Verification items for the finished model (mm, model axes). Face numbers are marked on the shaded views. A direction names the side the tool comes from. Give positions to 0.01 mm unless a question says otherwise; leave off trailing zeros. Write each loop counter-clockwise with the first axis right and the second up, starting at its lowest first coordinate (ties: lowest second). Pieces come first, ordered by that corner, then holes. Notation, with made-up numbers: (-16, -36.75) -> (31, -36.75) arc R13 cw to (31, -13.75) -> close; hole circle Ø11 at (72, 38.5). An arc over 180 degrees is marked (long way). Answer as CSV lines item,"result".
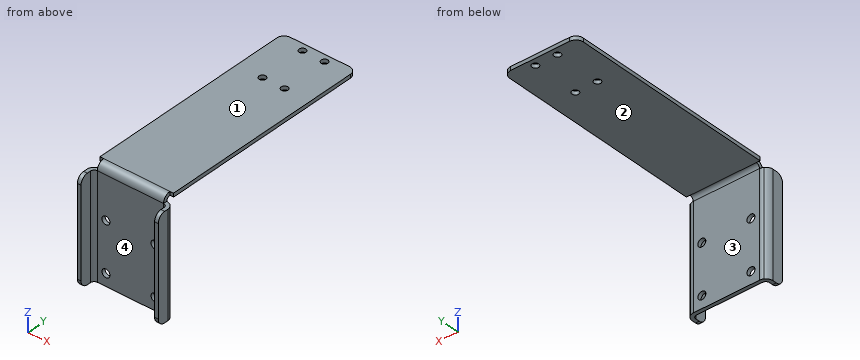
```python
from build123d import *

# Parameters (mm, degrees)
SKIZZE1_W                        = 60
SKIZZE1_H                        = 180
BASIS_BLECH1_DEPTH               = 3
KANTE_LASCHE1_STRIP_W            = 18
KANTE_LASCHE1_STRIP_H            = 3
KANTE_LASCHE1_STRIP_CUT_DEPTH    = 60
KANTE_LASCHE1_DEPTH              = 60
KANTE_LASCHE2_START              = -90.5
KANTE_LASCHE2_DEPTH              = 90.5
KANTE_LASCHE2_START_2            = -6
KANTE_LASCHE2_2_DEPTH            = 6
KANTE_LASCHE2_3_DEPTH            = 84.5
ECKE_START                       = -33
ECKE_BRECHEN1_DEPTH              = 66
ECKE_START_2                     = -3
ECKE_BRECHEN1_2_DEPTH            = 3
F_6_5_6_5_DURCHMESSER_BOHRUNG1_D = 6.5
F_5_5_5_5_DURCHMESSER_BOHRUNG1_D = 5.5


# Read off the part's stored shape, not the designer's step: Kante-Lasche2, Ecke brechen1
# Sheet-metal steps are written as plain solids
with BuildPart() as part:
    # Skizze1 → Basis-Blech1 (new body)
    with BuildSketch(Plane.XY):
        Rectangle(SKIZZE1_W, SKIZZE1_H)
    extrude(amount=-BASIS_BLECH1_DEPTH)

    # Kante-Lasche1 strip (across the edge) → Kante-Lasche1 strip cut (cut)
    with BuildSketch(Plane(origin=(30, -90, -3), x_dir=(0, 1, 0), z_dir=(-1, 0, 0))):
        with Locations((-3, -1.5)):
            Rectangle(KANTE_LASCHE1_STRIP_W, KANTE_LASCHE1_STRIP_H)
    extrude(amount=KANTE_LASCHE1_STRIP_CUT_DEPTH, mode=Mode.SUBTRACT)

    # Kante-Lasche1 section (across the edge) → Kante-Lasche1 (add)
    with BuildSketch(Plane(origin=(30, -90, -3), x_dir=(0, 1, 0), z_dir=(-1, 0, 0))):
        with BuildLine():
            Line((0, 3), (0, 87.5))
            Line((0, 87.5), (3, 87.5))
            Line((3, 87.5), (3, 3))
            ThreePointArc((3, 3), (3.878679656, 0.878679656), (6, 0))
            Line((6, 0), (6, -3))
            ThreePointArc((6, -3), (1.757359313, -1.242640687), (0, 3))
        make_face()
    extrude(amount=KANTE_LASCHE1_DEPTH)

    # Kante-Lasche2 outline → Kante-Lasche2 (cut)
    with BuildSketch(Plane.XY.offset(KANTE_LASCHE2_START)):
        with BuildLine():
            Line((-27, -87), (-27, -84))
            Line((-27, -84), (-30, -84))
            Line((-30, -84), (-30, -87.803847577))
            ThreePointArc((-30, -87.803847577), (-28.552914271, -87.204445042), (-27, -87))
        make_face()
        with BuildLine():
            Line((30, -84), (27, -84))
            Line((27, -84), (27, -87))
            ThreePointArc((27, -87), (28.552914271, -87.204445042), (30, -87.803847577))
            Line((30, -87.803847577), (30, -84))
        make_face()
    extrude(amount=KANTE_LASCHE2_DEPTH, mode=Mode.SUBTRACT)

    # Kante-Lasche2 2 outline → Kante-Lasche2 2 (cut)
    with BuildSketch(Plane.XY.offset(KANTE_LASCHE2_START_2)):
        with BuildLine():
            Line((-27, -90), (-27, -87))
            ThreePointArc((-27, -87), (-28.552914271, -87.204445042), (-30, -87.803847577))
            ThreePointArc((-30, -87.803847577), (-32.196152423, -90), (-33, -93))
            Line((-33, -93), (-33, -102))
            Line((-33, -102), (-30, -102))
            Line((-30, -102), (-30, -93))
            ThreePointArc((-30, -93), (-29.121320344, -90.878679656), (-27, -90))
        make_face()
        with BuildLine():
            ThreePointArc((30, -87.803847577), (28.552914271, -87.204445042), (27, -87))
            Line((27, -87), (27, -90))
            ThreePointArc((27, -90), (29.121320344, -90.878679656), (30, -93))
            Line((30, -93), (30, -102))
            Line((30, -102), (33, -102))
            Line((33, -102), (33, -93))
            ThreePointArc((33, -93), (32.196152423, -90), (30, -87.803847577))
        make_face()
    extrude(amount=KANTE_LASCHE2_2_DEPTH, mode=Mode.SUBTRACT)

    # Kante-Lasche2 3 outline → Kante-Lasche2 3 (add)
    with BuildSketch(Plane.XY.offset(KANTE_LASCHE2_START)):
        with BuildLine():
            Line((-27, -90), (-27, -87))
            ThreePointArc((-27, -87), (-28.552914271, -87.204445042), (-30, -87.803847577))
            ThreePointArc((-30, -87.803847577), (-32.196152423, -90), (-33, -93))
            Line((-33, -93), (-33, -102))
            Line((-33, -102), (-30, -102))
            Line((-30, -102), (-30, -93))
            ThreePointArc((-30, -93), (-29.121320344, -90.878679656), (-27, -90))
        make_face()
        with BuildLine():
            ThreePointArc((30, -87.803847577), (28.552914271, -87.204445042), (27, -87))
            Line((27, -87), (27, -90))
            ThreePointArc((27, -90), (29.121320344, -90.878679656), (30, -93))
            Line((30, -93), (30, -102))
            Line((30, -102), (33, -102))
            Line((33, -102), (33, -93))
            ThreePointArc((33, -93), (32.196152423, -90), (30, -87.803847577))
        make_face()
    extrude(amount=KANTE_LASCHE2_3_DEPTH)

    # Ecke brechen1 outline → Ecke brechen1 (cut)
    with BuildSketch(Plane.YZ.offset(ECKE_START)):
        with BuildLine():
            ThreePointArc((-96, -90.5), (-100.242640687, -88.742640687), (-102, -84.5))
            Line((-102, -84.5), (-102, -90.5))
            Line((-102, -90.5), (-96, -90.5))
        make_face()
        with BuildLine():
            ThreePointArc((-102, -12), (-100.242640687, -7.757359313), (-96, -6))
            Line((-96, -6), (-102, -6))
            Line((-102, -6), (-102, -12))
        make_face()
    extrude(amount=ECKE_BRECHEN1_DEPTH, mode=Mode.SUBTRACT)

    # Ecke brechen1 2 outline → Ecke brechen1 2 (cut)
    with BuildSketch(Plane.XY.offset(ECKE_START_2)):
        with BuildLine():
            Line((30, 90), (24, 90))
            ThreePointArc((24, 90), (28.242640687, 88.242640687), (30, 84))
            Line((30, 84), (30, 90))
        make_face()
        with BuildLine():
            ThreePointArc((-30, 84), (-28.242640687, 88.242640687), (-24, 90))
            Line((-24, 90), (-30, 90))
            Line((-30, 90), (-30, 84))
        make_face()
    extrude(amount=ECKE_BRECHEN1_2_DEPTH, mode=Mode.SUBTRACT)

    # Ø6.5 (6.5) Durchmesser Bohrung1 (through all)
    with Locations(Plane(origin=(0, -87, 0), x_dir=(1, 0, 0), z_dir=(0, 1, 0))):
        with Locations((-20, 80.5), (20, 80.5), (-20, 40.5), (20, 40.5)):
            Hole(F_6_5_6_5_DURCHMESSER_BOHRUNG1_D / 2)

    # Ø5.5 (5.5) Durchmesser Bohrung1 (through all)
    with Locations(Plane(origin=(0, 0, -3), x_dir=(-1, 0, 0), z_dir=(0, 0, -1))):
        with Locations((-9, 84), (9, 84), (-9, 46), (9, 46)):
            Hole(F_5_5_5_5_DURCHMESSER_BOHRUNG1_D / 2)


solid = part.part
```
1) Scan lines: line 1 along Z through (x, y) = (20, -88); line 2 along Z through (x, y) = (-20, -89); line 3 along Y through (x, z) = (9, -1). Record each from-to range of solid material in increasing order.
Reported:
line 1,"-90.5 to -83.75, -77.25 to -43.75, -37.25 to -1.53"
line 2,"-90.5 to -83.75, -77.25 to -43.75, -37.25 to -2.68"
line 3,"-87.32 to 43.25, 48.75 to 81.25, 86.75 to 90"
2) Depth check by flat-ended pin: pin 1 (12 mm diameter, centred on x = 16, y = 20, fed in from -Z); pin 2 (0.9 mm diameter, centred on y = -38, z = -2, fed in from +X); pin 3 (12 mm diameter, centred on x = 17, z = -13, fed in from +Y). Enter the tip coordinate at first touch or a pass-through.
Reported:
pin 1,"z = -3"
pin 2,"x = 30"
pin 3,"y = -87"
3) Section check B-B (x = 20). Record the boundary of the cut face in (y, z).
Reported:
outline,"(-90, -90.5) -> (-87, -90.5) -> (-87, -83.75) -> (-90, -83.75) -> close; (-90, -77.25) -> (-87, -77.25) -> (-87, -43.75) -> (-90, -43.75) -> close; (-90, -37.25) -> (-87, -37.25) -> (-87, -6) arc R3 cw to (-84, -3) -> (90, -3) -> (90, 0) -> (-84, 0) arc R6 ccw to (-90, -6) -> close"
4) Draft check along X on the marked faces 3 and 4. Enter one of: +X half, -X half, draft (parallel to the pull), parting line (faces both ways), or undercut.
Reported:
face 3,"draft"
face 4,"undercut"
5) Section check A-A (z = -80.5). Record the boundary of the cut face in (x, y).
Reported:
outline,"(-33, -102) -> (-30, -102) -> (-30, -93) arc R3 cw to (-27, -90) -> (-23.25, -90) -> (-23.25, -87) -> (-27, -87) arc R6 ccw to (-33, -93) -> close; (-16.75, -90) -> (16.75, -90) -> (16.75, -87) -> (-16.75, -87) -> close; (23.25, -90) -> (27, -90) arc R3 cw to (30, -93) -> (30, -102) -> (33, -102) -> (33, -93) arc R6 ccw to (27, -87) -> (23.25, -87) -> close"
6) Section check C-C (z = -64). Record the boundary of the cut face in (x, y).
Reported:
outline,"(-33, -102) -> (-30, -102) -> (-30, -93) arc R3 cw to (-27, -90) -> (27, -90) arc R3 cw to (30, -93) -> (30, -102) -> (33, -102) -> (33, -93) arc R6 ccw to (27, -87) -> (-27, -87) arc R6 ccw to (-33, -93) -> close"
7) Tool access check on the marked faces 1 and 2. Record the directions out of +Z, -Z, +X, -X, +Y, -Y that give a thin tool (end or side, any length) a straight path to the whole face; none if there is none.
Reported:
face 1,"+Z, +X, -X, +Y, -Y"
face 2,"-Z, +X, -X, +Y"
8) Section check D-D (x = -9). Record the boundary of the cut face in (y, z), and give its area (3 significant figures).
Reported:
outline,"(-90, -90.5) -> (-87, -90.5) -> (-87, -6) arc R3 cw to (-84, -3) -> (43.25, -3) -> (43.25, 0) -> (-84, 0) arc R6 ccw to (-90, -6) -> close; (48.75, -3) -> (81.25, -3) -> (81.25, 0) -> (48.75, 0) -> close; (86.75, -3) -> (90, -3) -> (90, 0) -> (86.75, 0) -> close"
area,"764 mm²"
